Answer from the drawing. Dimensions are ordinates in mm from the lowest x, y and z of the part. A direction names the side the tool comes from. Give positions to 0.01 mm unless a question says otherwise; leave off trailing zeros. Write each loop counter-clockwise with the first axis right and the second up, starting at its lowest first coordinate (ties: lowest second). Pieces come first, ordered by that corner, then holes.
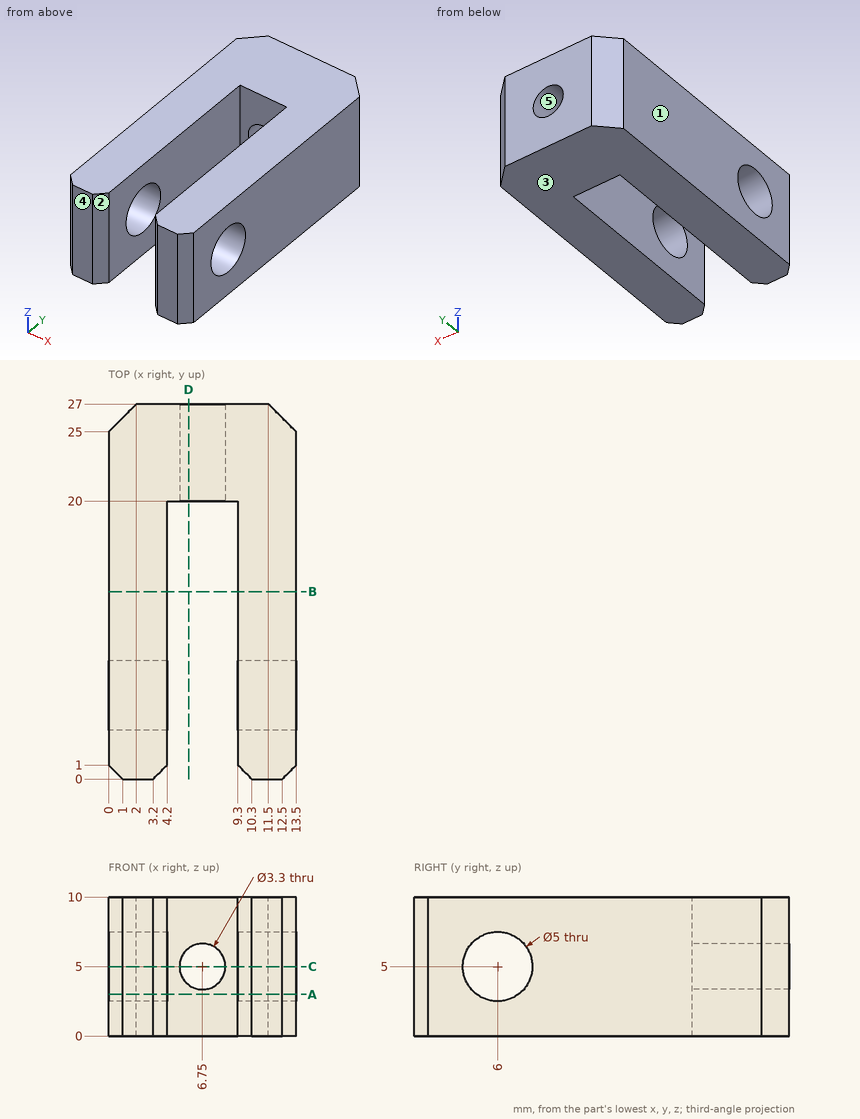
Item 1: Which of the six approach directions +Z, -Z, +X, -X, +Y, -Y give full straight-line access (tool end or side, diameter ignored) to the marked faces 1 and 2?
Result set:
face 1: +Z, -Z, -X, +Y, -Y
face 2: +Z, -Z, -Y
Item 2: Determine the mould class of the marked faces 3, 4 and 5 for opening direction Z: pulls with the +Z half, pulls with the -Z half, needs draft (parallel to the pull), parting line crosses it, or undercut.
Result set:
face 3: pulls with the -Z half
face 4: needs draft
face 5: undercut
Item 3: Section C-C (z = 5) is taken. Write down the section's boundary in (x, y).
Result set:
outline: (0, 1) - (1, 0) - (3.2, 0) - (4.2, 1) - (4.2, 3.5) - (0, 3.5) - close; (0, 8.5) - (4.2, 8.5) - (4.2, 20) - (5.1, 20) - (5.1, 27) - (2, 27) - (0, 25) - close; (8.4, 20) - (9.3, 20) - (9.3, 8.5) - (13.5, 8.5) - (13.5, 25) - (11.5, 27) - (8.4, 27) - close; (9.3, 1) - (10.3, 0) - (12.5, 0) - (13.5, 1) - (13.5, 3.5) - (9.3, 3.5) - close
Item 4: Section A-A (z = 3) is taken. Write down the section's boundary in (x, y).
Result set:
outline: (0, 1) - (1, 0) - (3.2, 0) - (4.2, 1) - (4.2, 4.5) - (0, 4.5) - close; (0, 7.5) - (4.2, 7.5) - (4.2, 20) - (9.3, 20) - (9.3, 7.5) - (13.5, 7.5) - (13.5, 25) - (11.5, 27) - (2, 27) - (0, 25) - close; (9.3, 1) - (10.3, 0) - (12.5, 0) - (13.5, 1) - (13.5, 4.5) - (9.3, 4.5) - close
Item 5: Find the intervals of material crossed by line 1 along X through (y, z) = (17.75, 7); line 2 along Y through (x, z) = (2.5, 5); line 3 along Z through (x, y) = (6.75, 22.75), in increasing order.
Result set:
line 1: x = 0 to 4.2, 9.3 to 13.5
line 2: y = 0 to 3.5, 8.5 to 27
line 3: z = 0 to 3.35, 6.65 to 10
Item 6: Section D-D (x = 5.75) is taken. Write down the section's boundary in (y, z), and give its area (3 significant figures).
Result set:
outline: (20, 0) - (27, 0) - (27, 3.69) - (20, 3.69) - close; (20, 6.31) - (27, 6.31) - (27, 10) - (20, 10) - close
area: 51.6 mm2
Item 7: Each of these flat-tipped pins is pushed along its axis until it touches: pin 1 Ø4.5 at (x, z) = (6.75, 5) entering from -Y; pin 2 Ø4 at (x, z) = (8, 5) entering from -Y. Where does it stop, or does it pass through?
Result set:
pin 1: stops at y = 20
pin 2: stops at y = 0.3
Item 8: Section B-B (y = 13.5) is taken. Write down the section's boundary in (x, z).
Result set:
outline: (0, 0) - (4.2, 0) - (4.2, 10) - (0, 10) - close; (9.3, 0) - (13.5, 0) - (13.5, 10) - (9.3, 10) - close
